```python
from build123d import *

# Parameters (mm, degrees)
F1_W     = 675
F1_H     = 460
F2_DEPTH = 690
F3_W     = 575
F3_H     = 360
F4_DEPTH = 110


with BuildPart() as f2:
    # F1 (on offset) → F2 (new body, through all)
    with BuildSketch(Plane.XY.offset(800)):
        with Locations((337.5, 230)):
            Rectangle(F1_W, F1_H)
    extrude(amount=-F2_DEPTH)

    # F3 (on face) → F4 (join, through all)
    with BuildSketch(Plane(origin=(0, 0, 110), x_dir=(1, 0, 0), z_dir=(0, 0, -1))):
        with Locations((337.5, -230)):
            Rectangle(F3_W, F3_H)
    extrude(amount=F4_DEPTH)


solid = f2.part
```
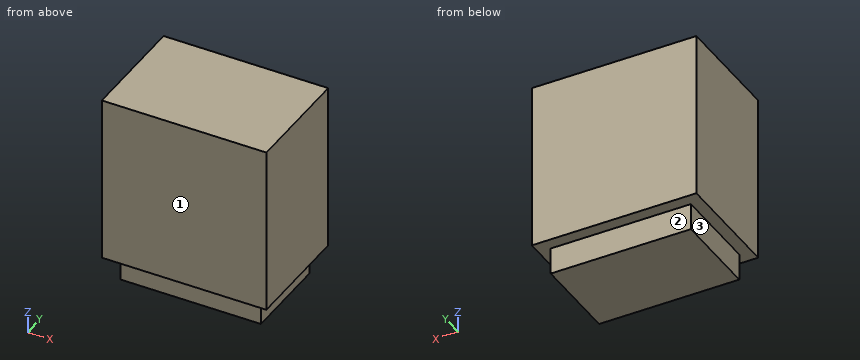
Can you work these out from the model? Positions are in its coordinate system, mm. Face numbers are marked on the shaded views. A direction names the side the tool comes from. Give positions to 0.01 mm unless a question says otherwise; leave off trailing zeros. Write each loop counter-clockwise with the first axis right and the second up, starting at its lowest first coordinate (ties: lowest second). Pieces come first, ordered by that corner, then holes. Notation, with made-up numbers: (7, -18) -> (32, -18) arc R12 ccw to (32, 0) -> close; hole circle Ø1 at (63.25, 77). An arc over 180 degrees is marked (long way). One line per item, written item: value.
Q1. For P1, Ø10, axis at x = 176.5, z = 324, coming from the -Y side, with a flat end and sliding along its axis, tell me the tip position at first contact or that it passes through.
Results found:
P1: stops at y = 0
Q2. Please list where these lines run through material, in increasing order: line 1 (X direction, y = 216.5, z = 72.5); line 2 (Z direction, x = 357.5, y = 415.5). Write a range as [from, to].
Results found:
line 1: x = [50, 625]
line 2: z = [110, 800]
Q3. Imagine slicing it at B-B on x = 84. Please give me the cut outline in (y, z).
Results found:
outline: (0, 110) -> (50, 110) -> (50, 0) -> (410, 0) -> (410, 110) -> (460, 110) -> (460, 800) -> (0, 800) -> close
Q4. Imagine slicing it at A-A on y = 224. Please give me the cut outline in (x, z), and give its area (3 significant figures).
Results found:
outline: (0, 110) -> (50, 110) -> (50, 0) -> (625, 0) -> (625, 110) -> (675, 110) -> (675, 800) -> (0, 800) -> close
area: 529,000 mm^2
Q5. Which directions (+Z, -Z, +X, -X, +Y, -Y) give clear straight access to the entire face, cutting with the end or side of a thin tool? Please do the marked faces 1, 2 and 3.
Results found:
face 1: +Z, -Z, +X, -X, -Y
face 2: -Z, +X, -X, +Y
face 3: -Z, -X, +Y, -Y
